from build123d import *

# Parameters (mm, degrees)
F0_W     = 80.8908492327
F0_H     = 37.8762930632
F1_DEPTH = 22
F3_D     = 5
F3_DEPTH = 28
F3_TIP   = 1.5021515476
F4_T     = -2
F6_D     = 5.5
F6_DEPTH = 2
F6_TIP   = 1.6523667023


with BuildPart() as f1:
    # F0 (on Front) → F1 (new body)
    with BuildSketch(Plane.XZ):
        with Locations((40.4454246163, 18.9381465316)):
            Rectangle(F0_W, F0_H)
    extrude(amount=F1_DEPTH)

    # F3
    with Locations(Plane.XZ.offset(22)):
        with Locations((4, 33.8762930632), (4, 4), (76.8908492327, 4), (76.8908492327, 33.8762930632)):
            Hole(F3_D / 2, depth=F3_DEPTH)
            with Locations((0, 0, -(F3_DEPTH + F3_TIP / 2))):  # 118° drill point
                Cone(0, F3_D / 2, F3_TIP, mode=Mode.SUBTRACT)

    # F4
    f4_openings = [f1.faces().sort_by_distance(p)[0] for p in [
        (40.445425, -22, 18.938147),
    ]]
    offset(amount=F4_T, openings=f4_openings)

    # F6
    with Locations(Plane(origin=(0, 0, 0), x_dir=(-1, 0, 0), z_dir=(0, 1, 0))):
        with Locations((-76.8908492327, 33.8762930632), (-76.8908492327, 4), (-4, 4), (-4, 32.8762930632)):
            Hole(F6_D / 2, depth=F6_DEPTH)
            with Locations((0, 0, -(F6_DEPTH + F6_TIP / 2))):  # 118° drill point
                Cone(0, F6_D / 2, F6_TIP, mode=Mode.SUBTRACT)


solid = f1.part
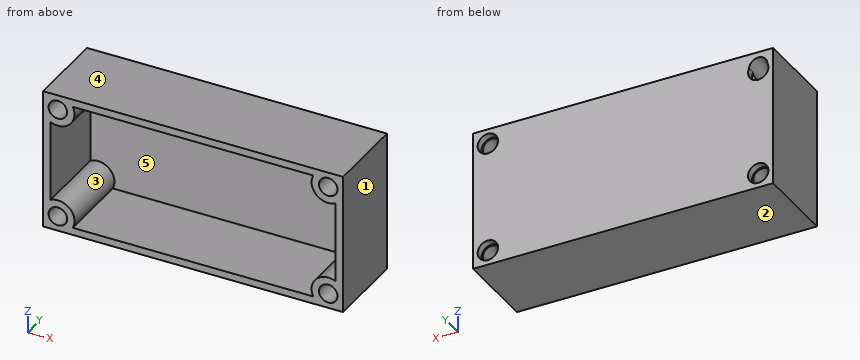
Check sheet for the modelled part. Datum: model origin and axes. Units: mm. Face numbers are marked on the shaded views. A direction names the side the tool comes from. Coordinates: 2 decimals unless noted, no trailing zeros. Write each loop counter-clockwise with the first axis right and the second up, starting at its lowest first coordinate (ties: lowest second). Pieces come first, ordered by that corner, then holes.
Item 1: Mould release check, pull along X, two halves, no side actions. Record for the marked faces 1, 2 and 3: released by +X, released by -X, zero draft, split by the parting line, or undercut.
Numbers:
face 1: released by +X
face 2: zero draft
face 3: undercut
Item 2: Access from +Z, -Z, +X, -X, +Y, -Y to the whole of each face (thin tool, end or side, straight path). Record for the marked faces 4 and 5.
Numbers:
face 4: +Z, +X, -X, +Y, -Y
face 5: -Y
Item 3: Cross-section at A-A on x = 4. Record the boundary of the cut face in (y, z).
Numbers:
outline: (-22, 0) - (0, 0) - (0, 1.25) - (-2, 1.25) - (-2.15, 1.5) - (-22, 1.5) - close; (-22, 6.5) - (-2.15, 6.5) - (-2, 6.75) - (0, 6.75) - (0, 30.13) - (-2, 30.13) - (-2.75, 31.38) - (-22, 31.38) - (-22, 29.38) - (-2, 29.38) - (-2, 8.5) - (-22, 8.5) - close; (-22, 36.38) - (0, 36.38) - (0, 37.88) - (-22, 37.88) - close
Item 4: Depth check by flat-ended pin: pin 1 Ø4 at (x, z) = (4, 33.88) entering from -Y; pin 2 Ø3.5 at (x, z) = (4, 32.88) entering from +Y; pin 3 Ø17 at (x, z) = (59, 19.5) entering from -Y. Enter the tip coordinate at first touch or a pass-through.
Numbers:
pin 1: passes through
pin 2: stops at y = -2.6
pin 3: stops at y = -2
Item 5: Cross-section at B-B on z = 4. Record the boundary of the cut face in (x, y), then the cut area to 3 significant figures.
Numbers:
outline: (0, -22) - (1.5, -22) - (1.5, -2.15) - (1.25, -2) - (1.25, 0) - (0, 0) - close; (6.5, -22) - (8.5, -22) - (8.5, -2) - (72.39, -2) - (72.39, -22) - (74.39, -22) - (74.39, -2.15) - (74.14, -2) - (74.14, 0) - (6.75, 0) - (6.75, -2) - (6.5, -2.15) - close; (79.39, -22) - (80.89, -22) - (80.89, 0) - (79.64, 0) - (79.64, -2) - (79.39, -2.15) - close
area: 280 mm2
Item 6: Scan lines: probe 1 along Z at (x, y) = (4, -9.5); probe 2 along X at (y, z) = (-0.8, 4); probe 3 along X at (y, z) = (-16, 4). Record each from-to range of solid material in increasing order.
Numbers:
probe 1: z = 0 to 1.5, 6.5 to 8.5, 29.38 to 31.38, 36.38 to 37.88
probe 2: x = 0 to 1.25, 6.75 to 74.14, 79.64 to 80.89
probe 3: x = 0 to 1.5, 6.5 to 8.5, 72.39 to 74.39, 79.39 to 80.89
Item 7: Cross-section at D-D on x = 39. Record the boundary of the cut face in (y, z).
Numbers:
outline: (-22, 0) - (0, 0) - (0, 37.88) - (-22, 37.88) - (-22, 35.88) - (-2, 35.88) - (-2, 2) - (-22, 2) - close
Item 8: Cross-section at C-C on z = 17.5. Record the boundary of the cut face in (x, y).
Numbers:
outline: (0, -22) - (2, -22) - (2, -2) - (78.89, -2) - (78.89, -22) - (80.89, -22) - (80.89, 0) - (0, 0) - close
